from build123d import *

# Parameters (mm, degrees)
SKETCH1_R             = 15
SKETCH1_R_2           = 23.5
BOSS_EXTRUDE1_DEPTH   = 12.7
M3X0_5_TAPPED_HOLE1_D = 2.5
M4X0_7_TAPPED_HOLE1_D = 3.3


with BuildPart() as part:
    # Sketch1 → Boss-Extrude1 (new body)
    with BuildSketch(Plane.XY.offset(12.7)):
        with BuildLine():
            Line((30, 23.323807579), (30, 305))
            ThreePointArc((30, 305), (0, 335), (-30, 305))
            Line((-30, 305), (-30, 23.323807579))
            ThreePointArc((-30, 23.323807579), (0, -38), (30, 23.323807579))
        make_face()
        with Locations(Location((0, 0, 0), (0, 0, 180))):
            Circle(SKETCH1_R, mode=Mode.SUBTRACT)
        with Locations(Location((0, 305, 0), (0, 0, 180))):
            Circle(SKETCH1_R_2, mode=Mode.SUBTRACT)
        with BuildLine():
            Line((18.5, 84.022471071), (18.5, 74.022471071))
            ThreePointArc((18.5, 74.022471071), (0, 55.522471071), (-18.5, 74.022471071))
            Line((-18.5, 74.022471071), (-18.5, 84.022471071))
            ThreePointArc((-18.5, 84.022471071), (0, 102.522471071), (18.5, 84.022471071))
        make_face(mode=Mode.SUBTRACT)
    extrude(amount=-BOSS_EXTRUDE1_DEPTH)

    # M3x0.5 Tapped Hole1 (through all)
    with Locations(Plane.XY.offset(12.7)):
        with Locations((0, 331.75), (3.299999999, 331.545668196), (23.166179551, 318.375), (26.749999999, 305), (23.166179551, 291.625), (0, 278.25), (-23.166179551, 291.625), (-26.750000001, 305), (-23.166179551, 318.375), (-3.300000001, 331.545668196), (26.749999999, 249.511235535), (21.578861519, 245.43367635), (1.619921459, 231.265288591), (-26.750000001, 249.511235535), (-26.750000001, 192.911235535), (-26.75, 186.111235535), (26.749999999, 192.911235535), (26.75, 186.111235535), (-26.75, 129.511235535), (26.75, 129.511235535), (-26.75, 74.022471071), (-3.3, 47.476802874), (3.4, 47.489425637), (26.75, 74.022471071)):
            Hole(M3X0_5_TAPPED_HOLE1_D / 2)

    # M4x0.7 Tapped Hole1 (through all)
    with Locations(Plane(origin=(0, 20.4, 12.7), x_dir=(1, 0, 0), z_dir=(0, 0, 1))):
        with Locations((0, 0), (14.424978336, -5.975021664), (20.4, -20.4), (14.424978336, -34.824978336), (0, -40.8), (-14.424978336, -34.824978336), (-20.4, -20.4), (-14.424978336, -5.975021664), (25.5016, 46.372471071), (25.5016, 70.872471071), (-25.5016, 70.872471071), (-25.5016, 46.372471071)):
            Hole(M4X0_7_TAPPED_HOLE1_D / 2)


solid = part.part
Can you work these out from the model? Positions are in its coordinate system, mm. A direction names the side the tool comes from. Give positions to 0.01 mm unless a question says otherwise; leave off trailing zeros. Loops run counter-clockwise (first coordinate to the right, second up) from the corner with the lowest first, then second, coordinate; pieces in that order, holes last. Notation, with made-up numbers: (81, -20.5) - (96, -20.5) arc R3 ccw to (96, -15.5) - close; hole circle Ø1 at (1, 67.5). An arc over 180 degrees is marked (long way). Return JSON: item names as keys, results as strings.
1. I'm going to push flat-ended pins straight in: pin 1 Ø3 at (y, z) = (212, 10) entering from +X; pin 2 Ø2.5 at (x, y) = (-14.42, 14.42) entering from +Z; pin 3 Ø3 at (y, z) = (217, 3) entering from -X; pin 4 Ø1.5 at (x, z) = (-4.5, 10.5) entering from -Y. Where does each tip first touch, or does it pass through?
Output values:
{"pin 1": "stops at x = 30", "pin 2": "passes through", "pin 3": "stops at x = -30", "pin 4": "stops at y = -37.81"}
2. I want a section at B-B on z = 9.5. Give the number of separate pieces and of enclosed holes in the cut face, and give its area (3 significant figures).
Output values:
{"separate pieces": "1", "enclosed holes": "39", "area": "18,100 mm²"}
3. I want a section at A-A on y = 149. Please give me the cut outline in (x, z), and give its area (3 significant figures).
Output values:
{"outline": "(-30, 0) - (30, 0) - (30, 12.7) - (-30, 12.7) - close", "area": "762 mm²"}
4. For faces 5 (the face through (-1, 151, 0)), 6 (the face through (-30, 166, 6)), 7 (the face through (-18.5, 79, 6)), which set-ups out of +Z, -Z, +X, -X, +Y, -Y let a thin tool reach every point of the face, with its end or its side?
Output values:
{"face 5": "-Z, +X, -X, +Y, -Y", "face 6": "+Z, -Z, -X, +Y", "face 7": "+Z, -Z"}
5. If I drill on line 1 (X direction, y = 250, z = 6.5); line 2 (X direction, y = 304, z = 3); line 3 (Y direction, x = -9, z = 7), over which ranges is the centre line in solid material (lowest first)?
Output values:
{"line 1": "x = -30 to -27.9, -25.6 to 25.6, 27.9 to 30", "line 2": "x = -30 to -27.5, -26 to -23.48, 23.48 to 26, 27.5 to 30", "line 3": "y = -36.92 to -12, 12 to 57.86, 100.19 to 283.29, 326.71 to 333.62"}
6. We'd pull the mould along Y, two halves only. Please class faces 1 (the face through (0.407, 55.527, 6.439)), 2 (the face through (0.66, 334.993, 6.439)), 3 (the face through (-0.407, 102.518, 6.439)), 4 (the face through (30, 162, 6)): +Y half, -Y half, draft (parallel to the pull), parting line (faces both ways), or undercut.
Output values:
{"face 1": "undercut", "face 2": "+Y half", "face 3": "undercut", "face 4": "draft"}
